Autodesk Inventor part; units mm, degrees
ref_plane "Work Plane1" through (0, 7, 0) normal (0, 1, 0) x (1, 0, 0)
ref_plane "Work Plane2" through (-0.7457, 7, -1.8253) normal (0.0048553, 0, -0.9999882) x (-0.9999882, 0, -0.0048553)
ref_plane "Work Plane3" through (0, 9, 0) normal (0, 1, 0) x (1, 0, 0)
ref_plane "Work Plane1" through (0, 7, 0) normal (0, 1, 0) x (1, 0, 0)
sketch "Sketch3" plane through (0, 7, 0) normal (0, 1, 0) x (1, 0, 0)
  line L0 (1.8253, 0.7457) -> (1.818, -0.7634)
  line L1 (1.818, -0.7634) -> (0.7457, -1.8253)
  line L2 (0.7457, -1.8253) -> (-0.7634, -1.818)
  line L3 (-0.7634, -1.818) -> (-1.8253, -0.7457)
  line L4 (-1.8253, -0.7457) -> (-1.818, 0.7634)
  line L5 (-1.818, 0.7634) -> (-0.7457, 1.8253)
  line L6 (-0.7457, 1.8253) -> (0.7634, 1.818)
  line L7 (0.7634, 1.818) -> (1.8253, 0.7457)
  line L8 (-1.8216, 0.0088) -> (1.8216, -0.0088) construction
  line L9 (-0.0088, -1.8216) -> (0.0088, 1.8216) construction
  point P0 (0, 0)
  point P1 (0, 0)
  point P2 (0, 0)
  point P3 (0, 0)
extrude "Extrusion2" add sketch "Sketch3" along normal blind 2
ref_plane "Work Plane2" through (-0.7457, 7, -1.8253) normal (0.0048553, 0, -0.9999882) x (-0.9999882, 0, -0.0048553)
sketch "Sketch4" plane through (-0.7457, 7, -1.8253) normal (0.0048553, 0, -0.9999882) x (-0.9999882, 0, -0.0048553)
  line L0 (-1.5091, 2) -> (0, 2)
  line L1 (0, 2) -> (0, 0)
  line L2 (0, 0) -> (-1.5091, 0)
  line L3 (-1.5091, 0) -> (-1.5091, 2)
  point P0 (-0.7546, -7)
extrude "Extrusion3" add sketch "Sketch4" along normal blind 10
sketch "Sketch5" plane through (0, 9, 0) normal (0, 1, 0) x (1, 0, 0)
  point P0 (0, 0)
sketch "Sketch6" plane through (0, 9, 0) normal (0, 1, 0) x (1, 0, 0)
  point P0 (0, 0)
sketch "Sketch7" plane through (0, 9, 0) normal (0, 1, 0) x (1, 0, 0)
  circle A0 centre (0.062, 12.7642) radius 1.2414
  point P0 (0, 0)
extrude "Extrusion4" add sketch "Sketch7" against normal blind 2
sketch "Sketch8" plane through (0, 9, 0) normal (0, 1, 0) x (1, 0, 0)
  point P0 (0, 0)
sketch "Sketch9" plane through (0, 9, 0) normal (0, 1, 0) x (1, 0, 0)
  point P0 (0, 0)
sketch "Sketch11" plane through (0, 9, 0) normal (0, 1, 0) x (1, 0, 0)
  point P0 (0, 0)
sketch "Sketch12" plane through (0, 9, 0) normal (0, 1, 0) x (1, 0, 0)
  point P0 (0, 0)
ref_plane "Work Plane3" through (0, 9, 0) normal (0, 1, 0) x (1, 0, 0)
sketch "Sketch13" plane through (0, 9, 0) normal (0, 1, 0) x (1, 0, 0)
  line L0 (0.062, 11.5229) -> (9.5019, 11.5229)
  line L1 (0.062, 11.5229) -> (0.062, 14.0056)
  arc A0 (0.8117, 11.7749) -> (-0.6974, 11.7822) centre (0.062, 12.7642) ccw
  line L2 (0.062, 14.0056) -> (9.5019, 14.0056)
  line L3 (9.5019, 11.5229) -> (9.5019, 14.0056)
  point P0 (0, 0)
extrude "Extrusion6" add sketch "Sketch13" against normal blind 2
ref_plane "Work Plane4" through (0, 9, 0) normal (0, 1, 0) x (1, 0, 0)
sketch "Sketch14" plane through (0, 9, 0) normal (0, 1, 0) x (1, 0, 0)
  line L0 (9.5019, 14.0056) -> (9.5019, 11.5229)
  circle A0 centre (9.5019, 12.7642) radius 1.2415
  point P0 (0, 0)
  dimension "d17" = 2.483
extrude "Extrusion7" add sketch "Sketch14" against normal blind 2
ref_plane "Work Plane5" through (0, 9, 0) normal (0, 1, 0) x (1, 0, 0)
sketch "Sketch15" plane through (0, 9, 0) normal (0, 1, 0) x (1, 0, 0)
  arc A0 (9.4834, 11.5229) -> (9.4834, 14.0056) centre (9.5019, 12.7642) ccw
  line L0 (10.7434, 12.7642) -> (13.7224, 9.3009)
  line L1 (9.4834, 11.5229) -> (11.3674, 9.2776)
  line L2 (9.4834, 11.5229) -> (12.4144, 11.5229) construction
  arc A1 (11.3674, 9.2776) -> (13.7224, 9.3009) centre (12.5353, 10.2576) ccw
  point P0 (0, 0)
  dimension "d20" = 50
extrude "Extrusion8" add sketch "Sketch15" against normal blind 2
sketch "Sketch16" plane through (0, 9, 0) normal (0, 1, 0) x (1, 0, 0)
  point P0 (0, 0)
hole "Hole1" at (0, 9, 0) direction (0, -1, 0) diameter 3 end through all
thread "Thread2"
fillet "Fillet1" radius 2 1 edges at (0.8105, 8, -11.5229)
fillet "Fillet2" radius 2 1 edges at (9.5019, 8, -11.5229)
fillet "Fillet3" radius 2 1 edges at (10.7434, 8, -12.7642)
properties part number "Servo_Arm_Hook_F"
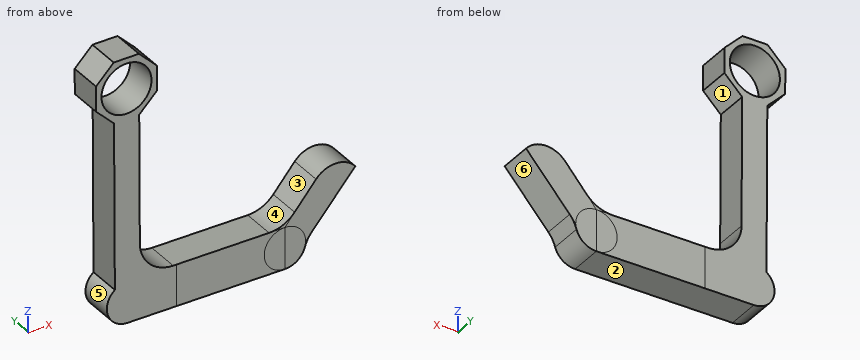
Geometry: final body of the model. Coordinates: model frame, mm. Face numbers are marked on the shaded views. A direction names the side the tool comes from. Round coordinates to 2 decimals unless told otherwise and drop trailing zeros. Loops run counter-clockwise (first coordinate to the right, second up) from the corner with the lowest first, then second, coordinate; pieces in that order, holes last.
Q1. Access query for the marked faces 1, 2 and 3. Directions: +Z, -Z, +X, -X, +Y, -Y. A direction counts if a zero-diameter tool reaches every point of the face in a straight line with its end or side. Return the directions, or none.
Q2. Pull-direction query (Z, two-part tool) for the marked faces 4, 5 and 6; classes: released by +Z, released by -Z, zero draft, split by the parting line, or undercut.
Q3. Material intervals for L1, parallel to Z at x = 0, y = 7.85; L2, parallel to X at y = 7.9, z = 0; L3, parallel to Z at x = -1, y = 8, sorted ascending.
Q4. Section B-B on y = 8.05. Return loops of the section in (x, z), plus the area to 3 significant figures.
Q5. Section A-A on z = -11. Return loops of the section in (x, y).
Q6. Pin query (flat end, axial travel): P1, Ø8, axis at x = 6.5, z = -9.5, coming from the -Y side; P2, Ø1, axis at y = 8, z = -4.5, coming from the -X side; P3, Ø0.6, axis at x = 5, y = 8.5, coming from the +Z side. Return the tip coordinate at first contact, or that it passes through.
Q7. Section C-C on x = 5.5. Return loops of the section in (y, z), plus the area to 3 significant figures.
Q8. Section D-D on z = 0. Return loops of the section in (x, y).
Evaluation:
1. face 1: +X, +Y, -Y
1. face 2: -Z, +X, -X, +Y, -Y
1. face 3: +Z, +Y, -Y
2. face 4: released by +Z
2. face 5: undercut
2. face 6: released by -Z
3. L1: z = -14 to -1.5, 1.5 to 1.82
3. L2: x = -1.82 to -1.5, 1.5 to 1.82
3. L3: z = -13.41 to -12.12, -1.57 to -1.12, 1.12 to 1.58
4. outline: (-1.83, 0.75) - (-1.82, -0.76) - (-0.75, -1.83) - (-0.7, -11.78) arc R1.24 ccw to (0.06, -14.01) - (9.5, -14.01) arc R1.24 ccw to (10.7, -13.1) arc R2 cw to (11.1, -12.34) - (13.72, -9.3) arc R1.52 ccw to (11.37, -9.28) - (10.08, -10.81) arc R2 cw to (8.55, -11.52) - (2.8, -11.52) arc R2 cw to (0.8, -9.53) - (0.76, -1.82) - (1.83, -0.75) - (1.82, 0.76) - (0.75, 1.83) - (-0.76, 1.82) - close; hole circle Ø3 at (0, 0)
4. area: 55.1 mm2
5. outline: (-0.7, 7) - (1.45, 7) - (1.45, 9) - (-0.7, 9) - close; (9.9, 7) - (12.26, 7) - (12.26, 9) - (9.9, 9) - close
6. P1: stops at y = 7
6. P2: stops at x = -0.74
6. P3: stops at z = -11.52
7. outline: (7, -14.01) - (9, -14.01) - (9, -11.52) - (7, -11.52) - close
7. area: 4.97 mm2
8. outline: (-1.82, 7) - (-1.5, 7) - (-1.5, 9) - (-1.82, 9) - close; (1.5, 7) - (1.82, 7) - (1.82, 9) - (1.5, 9) - close
